Check sheet for the modelled part. Datum: model origin and axes. Units: mm. Face numbers are marked on the shaded views. Coordinates: 2 decimals unless noted, no trailing zeros. Loops run counter-clockwise (first coordinate to the right, second up) from the corner with the lowest first, then second, coordinate; pieces in that order, holes last. Notation, with made-up numbers: (-7.75, -2.75) -> (31.25, -2.75) arc R7 ccw to (31.25, 9.25) -> close; hole circle Ø6 at (48.5, -30.75). An arc over 180 degrees is marked (long way). Use CSV: the item, a comma, the result in double quotes.
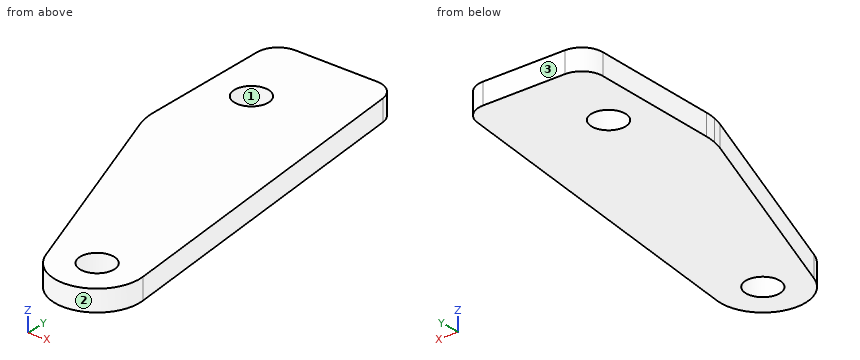
```python
from build123d import *

# Parameters (mm, degrees)
SZKIC1_R                    = 20
SZKIC1_R_2                  = 8
DODANIE_WYCI_GNI_CIE3_DEPTH = 10


with BuildPart() as part:
    # Szkic1 → Dodanie-wyciągnięcie3 (new body)
    # profile 1 of 3: a face of its own
    with BuildSketch(Plane.XY):
        with BuildLine():
            ThreePointArc((-57.25630176, 99), (-56.682391116, 96.462784094), (-55.890841639, 93.984823763))
            Line((-55.890841639, 93.984823763), (-18.769836395, -6.906029373))
            ThreePointArc((-18.769836395, -6.906029373), (-4.628612665, 19.457028159), (19.868958458, 2.285714286))
            Line((19.868958458, 2.285714286), (1.018920947, 166.142857143))
            ThreePointArc((1.018920947, 166.142857143), (-2.260807026, 172.464200273), (-8.915558282, 175))
            Line((-8.915558282, 175), (-17.736087047, 175))
            Line((-17.736087047, 175), (-17.736087047, 99))
            Line((-17.736087047, 99), (-57.25630176, 99))
        make_face()
    # profile 2 of 3: a face of its own
    with BuildSketch(Plane.XY):
        Circle(SZKIC1_R)
        Circle(SZKIC1_R_2, mode=Mode.SUBTRACT)
    # profile 3 of 3: a face of its own
    with BuildSketch(Plane.XY):
        with BuildLine():
            ThreePointArc((-57.736087047, 104.343867823), (-57.615899976, 101.661186457), (-57.25630176, 99))
            Line((-57.25630176, 99), (-17.736087047, 99))
            Line((-17.736087047, 99), (-17.736087047, 175))
            Line((-17.736087047, 175), (-47.736087047, 175))
            ThreePointArc((-47.736087047, 175), (-54.807154859, 172.071067812), (-57.736087047, 165))
            Line((-57.736087047, 165), (-57.736087047, 104.343867823))
        make_face()
        with Locations((-37.736087047, 137)):
            Circle(SZKIC1_R_2, mode=Mode.SUBTRACT)
    extrude(amount=DODANIE_WYCI_GNI_CIE3_DEPTH)


solid = part.part
```
1) Cross-section at A-A on z = 7. Record the boundary of the cut face in (x, y), and give its area (3 significant figures).
Answer below:
outline,"(-57.74, 104.34) arc R30 ccw to (-55.89, 93.98) -> (-18.77, -6.91) arc R20 ccw to (19.87, 2.29) -> (1.02, 166.14) arc R10 ccw to (-8.92, 175) -> (-47.74, 175) arc R10 ccw to (-57.74, 165) -> close; hole circle Ø16 at (-37.74, 137); hole circle Ø16 at (0, 0)"
area,"10,300 mm²"
2) Cross-section at B-B on x = -39. Record the boundary of the cut face in (y, z).
Answer below:
outline,"(48.08, 0) -> (129.1, 0) -> (129.1, 10) -> (48.08, 10) -> close; (144.9, 0) -> (175, 0) -> (175, 10) -> (144.9, 10) -> close"
3) Cross-section at C-C on y = 137. Record the boundary of the cut face in (x, z), and give its area (3 significant figures).
Answer below:
outline,"(-57.74, 0) -> (-45.74, 0) -> (-45.74, 10) -> (-57.74, 10) -> close; (-29.74, 0) -> (4.37, 0) -> (4.37, 10) -> (-29.74, 10) -> close"
area,"461 mm²"
4) Cross-section at D-D on y = 51.5. Record the boundary of the cut face in (x, z), and give its area (3 significant figures).
Answer below:
outline,"(-40.26, 0) -> (14.21, 0) -> (14.21, 10) -> (-40.26, 10) -> close"
area,"545 mm²"
5) Draft check along X on the marked faces 1, 2 and 3. Enter one of: released by +X, released by -X, zero draft, split by the parting line, or undercut.
Answer below:
face 1,"undercut"
face 2,"split by the parting line"
face 3,"zero draft"
6) Go/stop test with flat-tipped pins: pin 1 Ø9.5 at (x, y) = (0, 0) entering from +Z; pin 2 Ø6 at (x, z) = (-0.5, 2) entering from +Y. Record where each tip stops, or that it passes through.
Answer below:
pin 1,"passes through"
pin 2,"stops at y = 173.41"
7) Thickness scan on line 1 along Y through (x, z) = (-3, 4); line 2 along X through (y, z) = (2.5, 7.5); line 3 along X through (y, z) = (-5.5, 7.25). Record the ranges inside material, lowest first. Write a range as from..to.
Answer below:
line 1,"y = -19.77..-7.42, 7.42..173.06"
line 2,"x = -22.23..-7.6, 7.6..19.84"
line 3,"x = -19.29..-5.81, 5.81..19.23"
